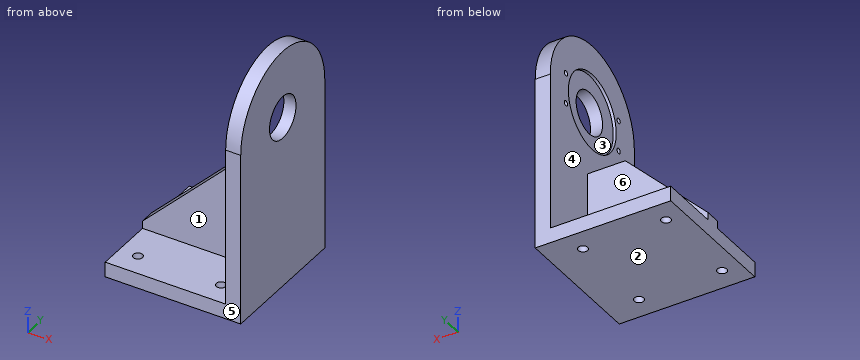
from build123d import *

# Parameters (mm, degrees)
F1_DEPTH       = 12.7
F2_D           = 36
F2_DEPTH       = 36
F2_CBORE_D     = 65
F2_CBORE_DEPTH = 2.5
F2_TIP         = 10.8154911425
F4_D           = 4.4
F4_DEPTH       = 10
F4_TIP         = 1.3218933619
F5_W           = 114.3
F5_H           = 12.7
F6_DEPTH       = 101.6
F7_W           = 101.6
F7_H           = 76.2
F8_DEPTH       = 6.35
F9_SIZE        = 69.85
F11_D          = 7.9375


# Not quite as in the source:
# - a length typed as a fraction of an inch, garbled in the dataset ("3 / 203.2 mm" for 3/8 in), is restored


with BuildPart() as f1:
    # F0 (on Right) → F1 (new body)
    with BuildSketch(Plane.YZ):
        with BuildLine():
            Line((57.15, -146.05), (57.15, 0))
            ThreePointArc((57.15, 0), (0, 57.15), (-57.15, 0))
            Line((-57.15, 0), (-57.15, -146.05))
            Line((-57.15, -146.05), (57.15, -146.05))
        make_face()
    extrude(amount=F1_DEPTH)

    # F2
    with Locations(Plane(origin=(0, 0, 0), x_dir=(0, 1, 0), z_dir=(-1, 0, 0))):
        with Locations((0, 0)):
            CounterBoreHole(F2_D / 2, F2_CBORE_D / 2, F2_CBORE_DEPTH, depth=F2_DEPTH)
            with Locations((0, 0, -(F2_DEPTH + F2_TIP / 2))):  # 118° drill point
                Cone(0, F2_D / 2, F2_TIP, mode=Mode.SUBTRACT)

    # F4
    with Locations(Plane(origin=(0, 0, 0), x_dir=(0, 1, 0), z_dir=(-1, 0, 0))):
        with Locations((35.814, -13.03522997), (35.814, 13.03522997), (-35.814, -13.03522997), (-35.814, 13.03522997)):
            Hole(F4_D / 2, depth=F4_DEPTH)
            with Locations((0, 0, -(F4_DEPTH + F4_TIP / 2))):  # 118° drill point
                Cone(0, F4_D / 2, F4_TIP, mode=Mode.SUBTRACT)

    # F5 (on face) → F6 (join)
    with BuildSketch(Plane.YZ):
        with Locations((0, -139.7)):
            Rectangle(F5_W, F5_H)
    extrude(amount=-F6_DEPTH)

    # F7 (on Front) → F8 (join, symmetric)
    with BuildSketch(Plane.XZ):
        with Locations((-50.8, -95.25)):
            Rectangle(F7_W, F7_H)
    extrude(amount=F8_DEPTH, both=True)

    # F9
    f9_edges = [f1.edges().sort_by_distance(p)[0] for p in [
        (-101.6, 0, -57.15),
    ]]
    chamfer(f9_edges, length=F9_SIZE)

    # F11 (through all)
    with Locations(Plane(origin=(0, 0, -146.05), x_dir=(1, 0, 0), z_dir=(0, 0, -1))):
        with Locations((-85.852, 38.1), (-15.748, 38.1), (-85.852, -38.1), (-15.748, -38.1)):
            Hole(F11_D / 2)


solid = f1.part
Build history of the part. All positions in model axes, mm. Face numbers are marked on the shaded views. A direction names the side the tool comes from. Give positions to 0.01 mm unless a question says otherwise; leave off trailing zeros. Loops run counter-clockwise (first coordinate to the right, second up) from the corner with the lowest first, then second, coordinate; pieces in that order, holes last. Notation, with made-up numbers: (20, 78) - (29, 78) arc R25 ccw to (29, 98) - close; hole circle Ø11 at (-8.5, -15). An arc over 180 degrees is marked (long way). Write item = value, one per line. Start each with the question number.
1) Pull direction Y, two halves, no side cores. Call the marked faces 3, 4, 5 and 6: +Y half, -Y half, draft (parallel to the pull), parting line (faces both ways), or undercut.
2) Band-saw the part on B-B on z = -60.5. Give the cut face in (x, y), plus the area to 3 significant figures.
3) Drop flat-ended pins along their axis: pin 1 Ø7 at (x, y) = (-15.748, 38.1) entering from +Z; pin 2 Ø10 at (x, y) = (-20.5, -2) entering from +Z; pin 3 Ø5.5 at (y, z) = (35.81, -13.04) entering from -X; pin 4 Ø4 at (x, y) = (-51, 6) entering from +Z. Give the stop position or say it passes through.
4) Probe probe 1 along X at (y, z) = (38, -136); probe 2 along Z at (x, y) = (-31, 1); probe 3 along Z at (x, y) = (-53.5, 41.5). List the from-to ranges inside material, lowest first. Write a range as from..to.
5) Band-saw the part on A-A on y = 0. Give the cut face in (x, z), plus the area to 3 significant figures.
6) Tool access for the marked faces 1 and 2: list every direction of +Z, -Z, +X, -X, +Y, -Y with a clear straight run to the whole face (end or side of a thin tool).
7) Band-saw the part on D-D on y = 46. Give the cut face in (x, z).
8) Band-saw the part on C-C on x = -93.5. Give the cut face in (y, z), plus the area to 3 significant figures.
Final values:
q1.face_3 = undercut
q1.face_4 = draft
q1.face_5 = -Y half
q1.face_6 = +Y half
q2.outline = (-35.1, -6.35) - (0, -6.35) - (0, -57.15) - (12.7, -57.15) - (12.7, 57.15) - (0, 57.15) - (0, 6.35) - (-35.1, 6.35) - close
q2.area = 1,900 mm²
q3.pin_1 = through
q3.pin_2 = -57.15
q3.pin_3 = 0
q3.pin_4 = -74.4
q4.probe_1 = -101.6..-89.82, -81.88..-19.72, -11.78..12.7
q4.probe_2 = -146.05..-57.15
q4.probe_3 = -146.05..-133.35
q5.outline = (-101.6, -146.05) - (12.7, -146.05) - (12.7, -18) - (2.5, -18) - (2.5, -32.5) - (0, -32.5) - (0, -57.15) - (-31.75, -57.15) - (-101.6, -127) - close; (0, 32.5) - (2.5, 32.5) - (2.5, 18) - (12.7, 18) - (12.7, 57.15) - (0, 57.15) - close
q5.area = 8,640 mm²
q6.face_1 = +Z, -X, -Y
q6.face_2 = -Z, +X, -X, +Y, -Y
q7.outline = (-101.6, -146.05) - (12.7, -146.05) - (12.7, 33.91) - (0, 33.91) - (0, -133.35) - (-101.6, -133.35) - close
q8.outline = (-57.15, -146.05) - (57.15, -146.05) - (57.15, -133.35) - (6.35, -133.35) - (6.35, -118.9) - (-6.35, -118.9) - (-6.35, -133.35) - (-57.15, -133.35) - close
q8.area = 1,640 mm²
